Check sheet for the modelled part. Datum: model origin and axes. Units: mm. Round coordinates to 2 decimals unless told otherwise and drop trailing zeros. Write each loop counter-clockwise with the first axis right and the second up, starting at its lowest first coordinate (ties: lowest second). Pieces come first, ordered by that corner, then holes.
Autodesk Inventor part; units mm, degrees
ref_plane "YZ Plane" through (0, 0, 0) normal (1, 0, 0) x (0, 1, 0)
ref_plane "XZ Plane" through (0, 0, 0) normal (0, 1, 0) x (-1, 0, 0)
ref_plane "XY Plane" through (0, 0, 0) normal (0, 0, 1) x (1, 0, 0)
sketch "Sketch1" plane through (0, 0, 0) normal (0, 1, 0) x (-1, 0, 0)
  line L0 (-40, -25) -> (40, -25)
  line L1 (35, 25) -> (-35, 25)
  line L2 (-49.8639, -13.356) -> (-44.8639, 16.644)
  line L3 (44.8639, 16.644) -> (49.8639, -13.356)
  circle A0 centre (-35, 15) radius 10
  circle A1 centre (-40, -15) radius 10
  circle A2 centre (35, 15) radius 10
  circle A3 centre (40, -15) radius 10
  line L4 (-35, 5) -> (35, 5)
  line L5 (-40, -5) -> (40, -5)
  line L6 (30.1361, -16.644) -> (25.1361, 13.356)
  line L7 (-25.1361, 13.356) -> (-30.1361, -16.644)
  point P0 (0, 0)
  point P1 (51.8046, -25)
  point P2 (0, 25)
  point P3 (0, -25)
  point P4 (0, -25)
  point P5 (-44.8639, 16.644)
  dimension "d22" = 70
  dimension "d23" = 50
  dimension "d24" = 25
  dimension "d25" = 80
  dimension "d26" = 20
extrude "Extrusion1" add sketch "Sketch1" along normal blind 5
hole "Hole2" at (-35, 0, 15) direction (0, 1, 0) diameter 9 end through all
pattern_sketch "Sketch Driven Pattern1" of "Hole2" from (-35, 0, 15) copies at (-40, 0, -15) at (40, 0, -15) at (35, 0, 15)
properties part number "PWTR-0085" material "Aluminum 6061"
1. Release check for a two-part mould opening along X. For faces 1 (the cylindrical face through (-30.61, 2.54, 15.98)), 2 (the cylindrical face through (-41, 2, 23)), 3 (the cylindrical face through (41.5, 2.5, 22.6)) record: released by +X, released by -X, zero draft, split by the parting line, or undercut.
2. Go/stop test with flat-tipped pins: pin 1 (1.5 mm diameter, centred on y = 4.5, z = 11, fed in from -X); pin 2 (10 mm diameter, centred on x = 28.5, z = -1, fed in from -Y); pin 3 (1.5 mm diameter, centred on x = -36, y = 4, fed in from +Z); pin 4 (1 mm diameter, centred on y = 1, z = -17.5, fed in from +X). Record where each tip stops, or that it passes through.
3. Scan lines: line 1 along X through (y, z) = (1.05, -15); line 2 along X through (y, z) = (3.35, 15); line 3 along Z through (x, y) = (35, 1.8). Record each from-to range of solid material in increasing order.
4. Sectioned sample at B-B, the plane y = 4. Enter the section's corners in (x, z), plus the area to 3 significant figures.
5. Sectioned sample at C-C, the plane z = 15. Enter the section's corners in (x, y).
6. Sectioned sample at D-D, the plane z = -2.5. Enter the section's corners in (x, y).
7. Sectioned sample at A-A, the plane z = -15. Enter the section's corners in (x, y), plus the area to 3 significant figures.
Computed values:
1. face 1: undercut
1. face 2: released by -X
1. face 3: released by +X
2. pin 1: stops at x = -45.93
2. pin 2: stops at y = 0
2. pin 3: stops at z = 25
2. pin 4: stops at x = 49.8
3. line 1: x = -50 to -44.5, -35.5 to 35.5, 44.5 to 50
3. line 2: x = -45.14 to -39.5, -30.5 to 30.5, 39.5 to 45.14
3. line 3: z = -25 to 10.5, 19.5 to 25
4. outline: (-49.86, -13.36) arc R10 ccw to (-40, -25) - (40, -25) arc R10 ccw to (49.86, -13.36) - (44.86, 16.64) arc R10 ccw to (35, 25) - (-35, 25) arc R10 ccw to (-44.86, 16.64) - close; hole circle Ø9 at (-40, -15); hole circle Ø9 at (-35, 15); hole circle Ø9 at (35, 15); hole circle Ø9 at (40, -15)
4. area: 4,420 mm2
5. outline: (-45.14, 0) - (-39.5, 0) - (-39.5, 5) - (-45.14, 5) - close; (-30.5, 0) - (30.5, 0) - (30.5, 5) - (-30.5, 5) - close; (39.5, 0) - (45.14, 0) - (45.14, 5) - (39.5, 5) - close
6. outline: (-48.05, 0) - (48.05, 0) - (48.05, 5) - (-48.05, 5) - close
7. outline: (-50, 0) - (-44.5, 0) - (-44.5, 5) - (-50, 5) - close; (-35.5, 0) - (35.5, 0) - (35.5, 5) - (-35.5, 5) - close; (44.5, 0) - (50, 0) - (50, 5) - (44.5, 5) - close
7. area: 410 mm2
